from build123d import *

# Parameters (mm, degrees)
SKIZZE1_R                                            = 2.5
AUFSATZ_LINEAR_AUSTRAGEN1_DEPTH                      = 5
STIRNSENKUNG_F_R_M3_ZYLINDERSCHRAUBE_MIT_D           = 3.4
STIRNSENKUNG_F_R_M3_ZYLINDERSCHRAUBE_MIT_CBORE_D     = 6.5
STIRNSENKUNG_F_R_M3_ZYLINDERSCHRAUBE_MIT_CBORE_DEPTH = 3.4


with BuildPart() as part:
    # Skizze1 → Aufsatz-Linear austragen1 (new body)
    with BuildSketch(Plane.XY):
        with BuildLine():
            Line((0, 0), (50, 0))
            Line((50, 0), (50, 45))
            ThreePointArc((50, 45), (45.606601718, 55.606601718), (35, 60))
            Line((35, 60), (15, 60))
            ThreePointArc((15, 60), (4.393398282, 55.606601718), (0, 45))
            Line((0, 45), (0, 0))
        make_face()
        with Locations((25, 45)):
            Circle(SKIZZE1_R, mode=Mode.SUBTRACT)
    extrude(amount=AUFSATZ_LINEAR_AUSTRAGEN1_DEPTH)

    # Stirnsenkung für M3 Zylinderschraube mit Innensechskant2 (through all)
    with Locations(Plane(origin=(0, 0, 0), x_dir=(-1, 0, 0), z_dir=(0, 0, -1))):
        with Locations((-40, 10), (-12, 10)):
            CounterBoreHole(STIRNSENKUNG_F_R_M3_ZYLINDERSCHRAUBE_MIT_D / 2, STIRNSENKUNG_F_R_M3_ZYLINDERSCHRAUBE_MIT_CBORE_D / 2, STIRNSENKUNG_F_R_M3_ZYLINDERSCHRAUBE_MIT_CBORE_DEPTH)


solid = part.part
Geometry: final body of the model. Coordinates: model frame, mm. A direction names the side the tool comes from. Coordinates: 2 decimals unless noted, no trailing zeros. Order: outer loops, then holes, each group sorted by start corner. A loop starts at its lowest first (then second) coordinate and runs counter-clockwise, first axis right, second up.
(1) Section query A-A (y = 10). Return the cut outline in (x, z), plus the area to 3 significant figures.
(2) Section query D-D (y = 54). Return the cut outline in (x, z), plus the area to 3 significant figures.
(3) First-contact query: pin 1 (4 mm diameter, centred on x = 12, y = 10, fed in from +Z); pin 2 (3 mm diameter, centred on x = 40, y = 8.5, fed in from -Z); pin 3 (3 mm diameter, centred on x = 25, y = 45, fed in from -Z); pin 4 (3 mm diameter, centred on x = 9.5, z = 2.5, fed in from +Y). Flat tips, straight axial feed; report the tip coordinate or a pass-through.
(4) Material intervals for probe 1 along Y at (x, z) = (25, 3.35); probe 2 along Y at (x, z) = (26.5, 2.85); probe 3 along X at (y, z) = (44.5, 3.3), sorted ascending.
(5) Section query B-B (x = 25). Return the cut outline in (y, z), plus the area to 3 significant figures.
(6) Section query C-C (z = 1.4). Return the cut outline in (x, y).
(7) Draft query along X for faces 1 (the face through (13.57, 9.35, 4.21)), 2 (the face through (45.72, 55.49, 2.46)), 3 (the face through (25, 60, 2)). Return one class per face: pulls with the +X half, pulls with the -X half, needs draft (parallel to the pull), parting line crosses it, or undercut.
(8) Access query for faces 4 (the face through (38.65, 8.97, 4.21)), 5 (the face through (38.6, 8.6, 3.4)). Directions: +Z, -Z, +X, -X, +Y, -Y. A direction counts if a zero-diameter tool reaches every point of the face in a straight line with its end or side. Return the directions, or none.
Solution:
1. outline: (0, 0) - (8.75, 0) - (8.75, 3.4) - (10.3, 3.4) - (10.3, 5) - (0, 5) - close; (13.7, 3.4) - (15.25, 3.4) - (15.25, 0) - (36.75, 0) - (36.75, 3.4) - (38.3, 3.4) - (38.3, 5) - (13.7, 5) - close; (41.7, 3.4) - (43.25, 3.4) - (43.25, 0) - (50, 0) - (50, 5) - (41.7, 5) - close
1. area: 195 mm2
2. outline: (3, 0) - (47, 0) - (47, 5) - (3, 5) - close
2. area: 220 mm2
3. pin 1: stops at z = 5
3. pin 2: stops at z = 3.4
3. pin 3: passes through
3. pin 4: stops at y = 59.46
4. probe 1: y = 0 to 42.5, 47.5 to 60
4. probe 2: y = 0 to 43, 47 to 60
4. probe 3: x = 0 to 22.55, 27.45 to 50
5. outline: (0, 0) - (42.5, 0) - (42.5, 5) - (0, 5) - close; (47.5, 0) - (60, 0) - (60, 5) - (47.5, 5) - close
5. area: 275 mm2
6. outline: (0, 0) - (50, 0) - (50, 45) arc R15 ccw to (35, 60) - (15, 60) arc R15 ccw to (0, 45) - close; hole circle Ø6.5 at (12, 10); hole circle Ø5 at (25, 45); hole circle Ø6.5 at (40, 10)
7. face 1: undercut
7. face 2: pulls with the +X half
7. face 3: needs draft
8. face 4: +Z, -Z
8. face 5: -Z
